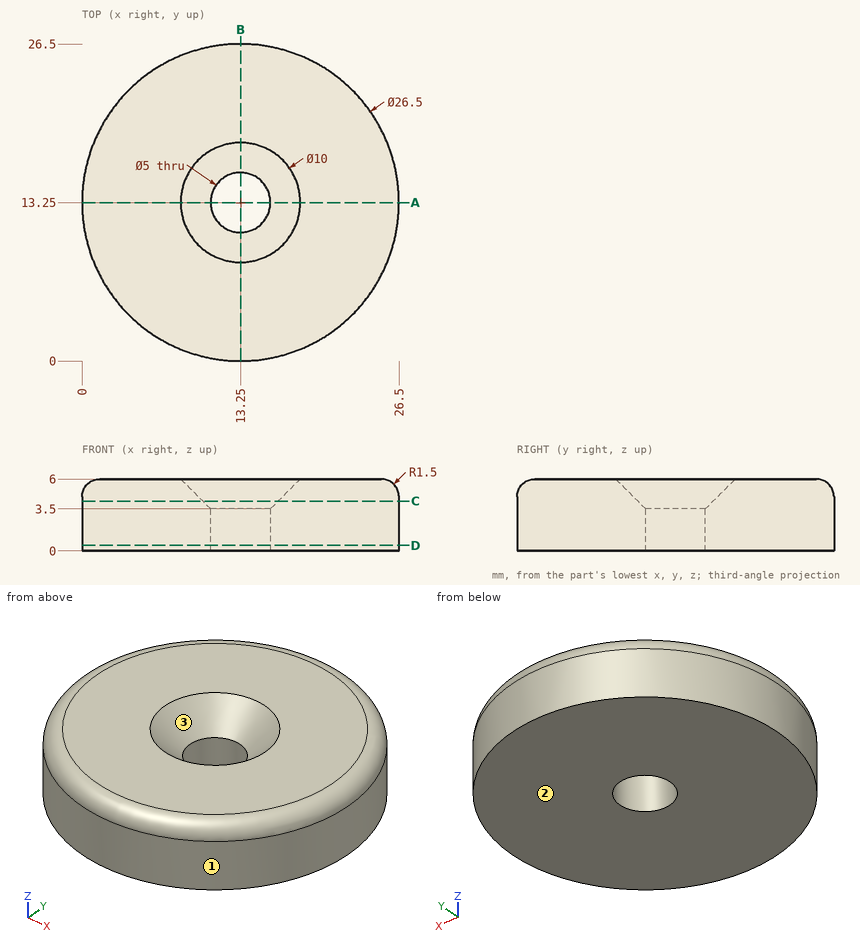
Here's the drawing with two shaded views (mm, measured from the low corner). I have some questions. Give positions to 0.01 mm unless a question says otherwise; leave off trailing zeros. Loops run counter-clockwise (first coordinate to the right, second up) from the corner with the lowest first, then second, coordinate; pieces in that order, holes last. Notation, with made-up numbers: (20, -27) -> (59, -27) arc R17 ccw to (59, -10) -> close; hole circle Ø5 at (-12.5, 26). An arc over 180 degrees is marked (long way). Answer as a JSON object with one key per item and string values. Group by question number.
Item 1: I need wall thicknesses on L1, parallel to Y at x = 13.25, z = 2.3; L2, parallel to Y at x = 16.75, z = 5.2; L3, parallel to X at y = 8.5, z = 3.5. Which ranges of each line are inside material? Lowest first, please.
Item 2: Thinking about a two-plate mould opening in X: for the marked faces 1, 2 and 3, which applies, pulls with the +X half, pulls with the -X half, needs draft (parallel to the pull), parting line crosses it, or undercut?
Item 3: Imagine slicing it at D-D on z = 0.45. Write out the boundary of the cut face in (x, y).
Item 4: Imagine slicing it at C-C on z = 4.15. Write out the boundary of the cut face in (x, y), then the cut area to 3 significant figures.
Item 5: Will this pin go through, and if not, where does the flat tip stop? pin 1 (4 mm diameter, centred on x = 13.25, y = 13.25, fed in from +Z).
Item 6: Imagine slicing it at A-A on y = 13.25. Write out the boundary of the cut face in (x, z), then the cut area to 3 significant figures.
Answer list:
{
 "1": {"L1": "y = 0 to 10.75, 15.75 to 26.5", "L2": "y = 0.65 to 10.93, 15.57 to 25.85", "L3": "x = 0.88 to 25.62"},
 "2": {"face 1": "parting line crosses it", "face 2": "needs draft", "face 3": "undercut"},
 "3": {"outline": "circle Ø26.5 at (13.25, 13.25); hole circle Ø5 at (13.25, 13.25)"},
 "4": {"outline": "circle Ø26.5 at (13.25, 13.25); hole circle Ø6.3 at (13.25, 13.25)", "area": "520 mm2"},
 "5": {"pin 1": "passes through"},
 "6": {"outline": "(0, 0) -> (10.75, 0) -> (10.75, 3.5) -> (8.25, 6) -> (1.5, 6) arc R1.5 ccw to (0, 4.5) -> close; (15.75, 0) -> (26.5, 0) -> (26.5, 4.5) arc R1.5 ccw to (25, 6) -> (18.25, 6) -> (15.75, 3.5) -> close", "area": "122 mm2"}
}
